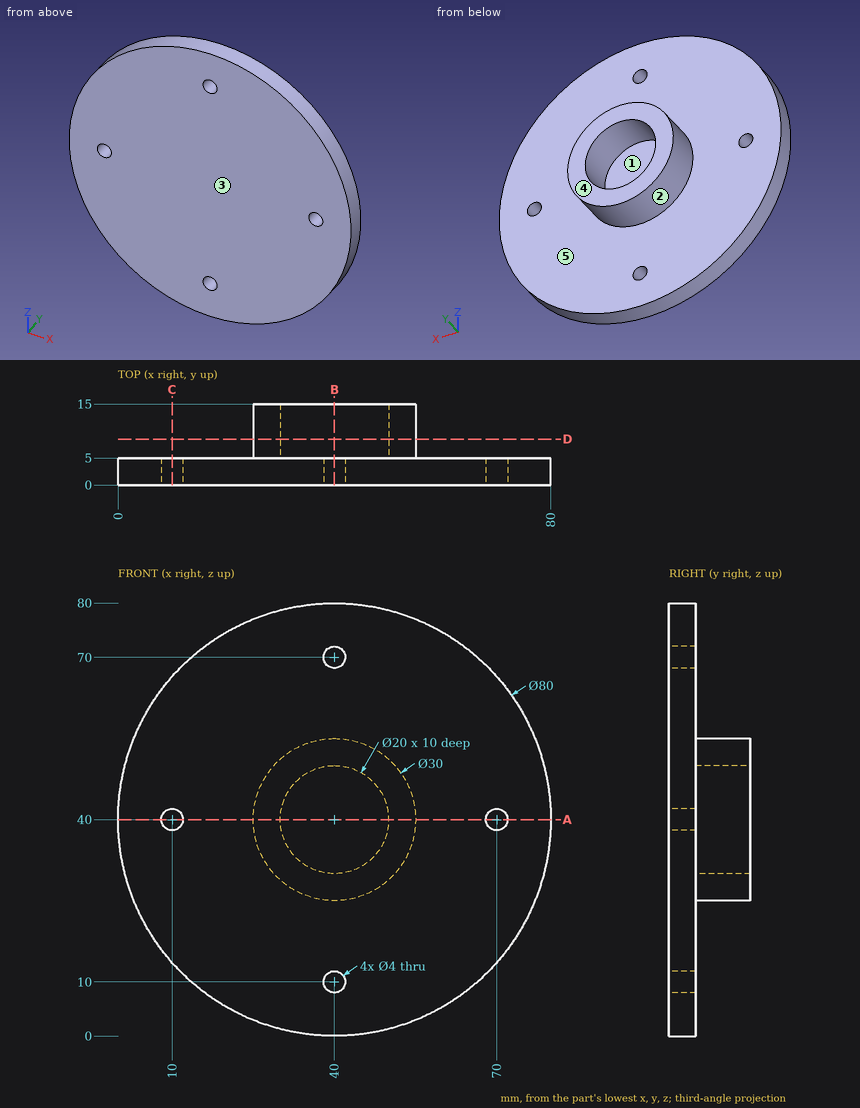
Could you check a few things on this drawing? It's one solid part, dimensions in mm from its lowest x, y, z. A direction names the side the tool comes from. Coordinates: 2 decimals unless noted, no trailing zeros. Order: outer loops, then holes, each group sorted by start corner. A loop starts at its lowest first (then second) coordinate and runs counter-clockwise, first axis right, second up.
1. For the marked faces 4 and 5, which set-ups out of +Z, -Z, +X, -X, +Y, -Y let a thin tool reach every point of the face, with its end or its side?
2. If we section it at B-B (x = 40): Please give me the cut outline in (y, z).
3. I need wall thicknesses on line 1 (X direction, y = 1.8, z = 40); line 2 (X direction, y = 10.5, z = 40); line 3 (Z direction, x = 16, y = 3.25). Which ranges of each line are inside material? Lowest first, please.
4. If we section it at C-C (x = 10): Please give me the cut outline in (y, z).
5. Thinking about a two-plate mould opening in Z: for the marked faces 1, 2 and 3, which applies, +Z half, -Z half, draft (parallel to the pull), parting line (faces both ways), or undercut?
6. I'm going to push flat-ended pins straight in: pin 1 (8 mm diameter, centred on x = 68.5, z = 49.5, fed in from +Y); pin 2 (6.5 mm diameter, centred on x = 70, z = 40, fed in from -Y); pin 3 (4 mm diameter, centred on y = 3.5, z = 25, fed in from +X); pin 4 (1 mm diameter, centred on y = 12, z = 33.5, fed in from -X). Where does each tip first touch, or does it pass through?
7. If we section it at D-D (y = 8.5): Please give me the cut outline in (x, z), then the cut area to 3 significant figures.
8. If we section it at A-A (z = 40): Please give me the cut outline in (x, y).
Entries:
1. face 4: +Z, -Z, +X, -X, +Y
1. face 5: +Y
2. outline: (0, 0) - (5, 0) - (5, 8) - (0, 8) - close; (0, 12) - (5, 12) - (5, 25) - (15, 25) - (15, 30) - (5, 30) - (5, 50) - (15, 50) - (15, 55) - (5, 55) - (5, 68) - (0, 68) - close; (0, 72) - (5, 72) - (5, 80) - (0, 80) - close
3. line 1: x = 0 to 8, 12 to 68, 72 to 80
3. line 2: x = 25 to 30, 50 to 55
3. line 3: z = 8 to 72
4. outline: (0, 13.54) - (5, 13.54) - (5, 38) - (0, 38) - close; (0, 42) - (5, 42) - (5, 66.46) - (0, 66.46) - close
5. face 1: undercut
5. face 2: parting line
5. face 3: draft
6. pin 1: stops at y = 5
6. pin 2: stops at y = 0
6. pin 3: stops at x = 77.83
6. pin 4: stops at x = 26.25
7. outline: circle Ø30 at (40, 40); hole circle Ø20 at (40, 40)
7. area: 393 mm2
8. outline: (0, 0) - (8, 0) - (8, 5) - (0, 5) - close; (12, 0) - (68, 0) - (68, 5) - (55, 5) - (55, 15) - (50, 15) - (50, 5) - (30, 5) - (30, 15) - (25, 15) - (25, 5) - (12, 5) - close; (72, 0) - (80, 0) - (80, 5) - (72, 5) - close
